Design review of the part built by this model. Coordinates are the model's own, in mm. A direction names the side the tool comes from. Give positions to 0.01 mm unless a question says otherwise; leave off trailing zeros. Write each loop counter-clockwise with the first axis right and the second up, starting at its lowest first coordinate (ties: lowest second). Pieces come first, ordered by that corner, then holes.
```python
from build123d import *

# Parameters (mm, degrees)
EXTRUDE_1_DEPTH          = 20
FILLET_1_R               = 4
SKETCH_3_W               = 42
SKETCH_3_H               = 4
EXTRUDE_2_DEPTH          = 42
FILLET_2_R               = 14
CHAMFER_1_SIZE           = 5
CUT_EXTRUDE_1_DEPTH      = 97.177520869
CUT_EXTRUDE_1_DEPTH_BACK = 97.177520869
SKETCH_2_R               = 2.8
SKETCH_2_R_2             = 2.3
SKETCH_2_R_3             = 11.5
SKETCH_2_R_4             = 1.8


with BuildPart() as part:
    # 草图1 → 凸台-拉伸1 (new body)
    with BuildSketch(Plane.XY):
        with BuildLine():
            Line((54.2, 3.8), (54.2, 0.2))
            Line((54.2, 0.2), (72.997777503, 0.2))
            Line((72.997777503, 0.2), (72.997777503, 4.2))
            Line((72.997777503, 4.2), (64.891608375, 4.2))
            ThreePointArc((64.891608375, 4.2), (60.821632223, 5.312671482), (57.883792669, 8.341176471))
            ThreePointArc((57.883792669, 8.341176471), (50, 13), (42.116207331, 8.341176471))
            ThreePointArc((42.116207331, 8.341176471), (39.178367777, 5.312671482), (35.108391625, 4.2))
            Line((35.108391625, 4.2), (-35.108391625, 4.2))
            ThreePointArc((-35.108391625, 4.2), (-39.178367777, 5.312671482), (-42.116207331, 8.341176471))
            ThreePointArc((-42.116207331, 8.341176471), (-50, 13), (-57.883792669, 8.341176471))
            ThreePointArc((-57.883792669, 8.341176471), (-60.821632223, 5.312671482), (-64.891608375, 4.2))
            Line((-64.891608375, 4.2), (-72.997777503, 4.2))
            Line((-72.997777503, 4.2), (-72.997777503, 0.2))
            Line((-72.997777503, 0.2), (-54.2, 0.2))
            Line((-54.2, 0.2), (-54.2, 3.8))
            ThreePointArc((-54.2, 3.8), (-50, 8), (-45.8, 3.8))
            Line((-45.8, 3.8), (-45.8, 0.2))
            Line((-45.8, 0.2), (45.8, 0.2))
            Line((45.8, 0.2), (45.8, 3.8))
            ThreePointArc((45.8, 3.8), (50, 8), (54.2, 3.8))
        make_face()
    extrude(amount=EXTRUDE_1_DEPTH)

    # 圆角1
    fillet_1_edges = [part.edges().sort_by_distance(p)[0] for p in [
        (72.997777503, 2.2, 20),
        (-72.997777503, 2.2, 0),
        (72.997777503, 2.2, 0),
        (-72.997777503, 2.2, 20),
    ]]
    fillet(fillet_1_edges, radius=FILLET_1_R)

    # 草图3 → 凸台-拉伸2 (add)
    with BuildSketch(Plane.XY.offset(20)):
        with Locations((0, 2.2)):
            Rectangle(SKETCH_3_W, SKETCH_3_H)
    extrude(amount=EXTRUDE_2_DEPTH)

    # 圆角2
    fillet_2_edges = [part.edges().sort_by_distance(p)[0] for p in [
        (-21, 2.2, 20),
        (21, 2.2, 20),
    ]]
    fillet(fillet_2_edges, radius=FILLET_2_R)

    # 倒角1
    chamfer_1_edges = [part.edges().sort_by_distance(p)[0] for p in [
        (-21, 2.2, 62),
        (21, 2.2, 62),
    ]]
    chamfer(chamfer_1_edges, length=CHAMFER_1_SIZE)

    # 草图2 → 切除-拉伸1 (cut, two sides: drawn at the far end of the back side and taken through both)
    with BuildSketch(Plane(origin=(0, 4.2, 0), x_dir=(1, 0, 0), z_dir=(0, 1, 0)).offset(-CUT_EXTRUDE_1_DEPTH_BACK)):
        with Locations(Location((0, -10, 0), (0, 0, 270))):
            Circle(SKETCH_2_R)
        with Locations(Location((67.197777503, -10, 0), (0, 0, 270))):
            Circle(SKETCH_2_R_2)
        with Locations(Location((32.802222497, -10, 0), (0, 0, 90))):
            Circle(SKETCH_2_R_2)
        with Locations(Location((-32.802222497, -10, 0), (0, 0, 270))):
            Circle(SKETCH_2_R_2)
        with Locations((-67.197777503, -10)):
            Circle(SKETCH_2_R_2)
        with Locations(Location((0, -41, 0), (0, 0, 270))):
            Circle(SKETCH_2_R_3)
        with Locations(Location((15.5, -25.5, 0), (0, 0, 270))):
            Circle(SKETCH_2_R_4)
        with Locations(Location((15.5, -56.5, 0), (0, 0, 270))):
            Circle(SKETCH_2_R_4)
        with Locations(Location((-15.5, -56.5, 0), (0, 0, 270))):
            Circle(SKETCH_2_R_4)
        with Locations(Location((-15.5, -25.5, 0), (0, 0, 270))):
            Circle(SKETCH_2_R_4)
    extrude(amount=CUT_EXTRUDE_1_DEPTH + CUT_EXTRUDE_1_DEPTH_BACK, mode=Mode.SUBTRACT)


solid = part.part
```
(1) Consider section A-A, the plane x = 0. Give the boundary of the cut face in (y, z), then the cut area to 3 significant figures.
Resolved:
outline: (0.2, 0) - (4.2, 0) - (4.2, 7.2) - (0.2, 7.2) - close; (0.2, 12.8) - (4.2, 12.8) - (4.2, 29.5) - (0.2, 29.5) - close; (0.2, 52.5) - (4.2, 52.5) - (4.2, 62) - (0.2, 62) - close
area: 134 mm2
(2) Tool access review of faces 4 (the face through (71.857, 2.228, 1.203)), 5 (the face through (-54.2, 2, 10)), 6 (the face through (-70, 4.2, 10)), 7 (the face through (70, 4.2, 10)), 8 (the face through (-21, 2, 45)): name each direction out of +Z, -Z, +X, -X, +Y, -Y from which nothing blocks a thin tool from reaching the whole face with its end or side.
Resolved:
face 4: -Z, +X, +Y, -Y
face 5: +Z, -Z, -Y
face 6: +Z, -Z, -X, +Y
face 7: +Z, -Z, +X, +Y
face 8: +Z, -X, +Y, -Y
(3) Consider section B-B, the plane z = 40. Give the boundary of the cut face in (x, y), then the cut area to 3 significant figures.
Resolved:
outline: (-21, 0.2) - (-11.46, 0.2) - (-11.46, 4.2) - (-21, 4.2) - close; (11.46, 0.2) - (21, 0.2) - (21, 4.2) - (11.46, 4.2) - close
area: 76.3 mm2
(4) Mouldability with a two-part tool opening along X and no side actions: class faces 1 (the face through (-39.127, 5.282, 9.86)), 2 (the face through (-64, 0.2, 10)), 3 (the face through (71.857, 2.228, 18.797)) as pulls with the +X half, pulls with the -X half, needs draft (parallel to the pull), parting line crosses it, or undercut.
Resolved:
face 1: undercut
face 2: needs draft
face 3: pulls with the +X half
(5) Consider section C-C, the plane y = 5.75. Give the boundary of the cut face in (x, z).
Resolved:
outline: (-60.16, 0) - (-53.72, 0) - (-53.72, 20) - (-60.16, 20) - close; (-46.28, 0) - (-39.84, 0) - (-39.84, 20) - (-46.28, 20) - close; (39.84, 0) - (46.28, 0) - (46.28, 20) - (39.84, 20) - close; (53.72, 0) - (60.16, 0) - (60.16, 20) - (53.72, 20) - close
(6) Clearance check with flat-ended pins moving along their axes: P1, Ø3, axis at y = 10, z = 7, coming from the +X side; P2, Ø5.5, axis at x = -67.2, z = 10, coming from the +Y side; P3, Ø2, axis at y = 9.5, z = 20, coming from the -X side. State where each tip first meets the part, or that it passes through.
Resolved:
P1: stops at x = 57.79
P2: stops at y = 4.21
P3: stops at x = -57.79
(7) To check wall thickness, follow L1, parallel to X at y = 3.35, z = 56.5; L2, parallel to X at y = 5, z = 5.5; L3, parallel to Z at x = -16.5, y = 1.5. State the ranges of each line that lie inside material, in increasing order.
Resolved:
L1: x = -21 to -17.3, -13.7 to 13.7, 17.3 to 21
L2: x = -61.4 to -54.02, -45.98 to -38.6, 38.6 to 45.98, 54.02 to 61.4
L3: z = 0 to 24, 27 to 55, 58 to 61.5
(8) Consider section D-D, the plane z = 10. Give the number of separate pieces and of enclosed holes in the cut face, then the cut area to 3 significant figures.
Resolved:
separate pieces: 6
enclosed holes: 0
area: 641 mm2
